Can you work these out from the model? Positions are in its coordinate system, mm. Coordinates: 2 decimals unless noted, no trailing zeros. Order: outer loops, then holes, each group sorted by start corner. A loop starts at its lowest first (then second) coordinate and runs counter-clockwise, first axis right, second up. Notation, with made-up numbers: (21.5, 18.5) -> (72.5, 18.5) arc R12 cw to (72.5, 40.5) -> close; hole circle Ø1 at (-35.5, 32.5). An arc over 180 degrees is marked (long way). Answer in a Markdown table with one row per item.
```python
from build123d import *

# Parameters (mm, degrees)
CYLINDER_R        = 35
CYLINDER_DEPTH    = 375
CYLINDER001_R     = 7.5
CYLINDER001_DEPTH = 390


with BuildPart() as part:
    # Cylinder → Cylinder (join)
    with BuildSketch(Plane.XY):
        Circle(CYLINDER_R)
    cylinder = extrude(amount=CYLINDER_DEPTH)

    # Cylinder001 → Cylinder001 (join)
    with BuildSketch(Plane.XY):
        Circle(CYLINDER001_R)
    cylinder001 = extrude(amount=CYLINDER001_DEPTH)

    # Mirrored001: Cylinder, Cylinder001 across XY
    add(cylinder.mirror(Plane.XY))
    add(cylinder001.mirror(Plane.XY))


solid = part.part
```
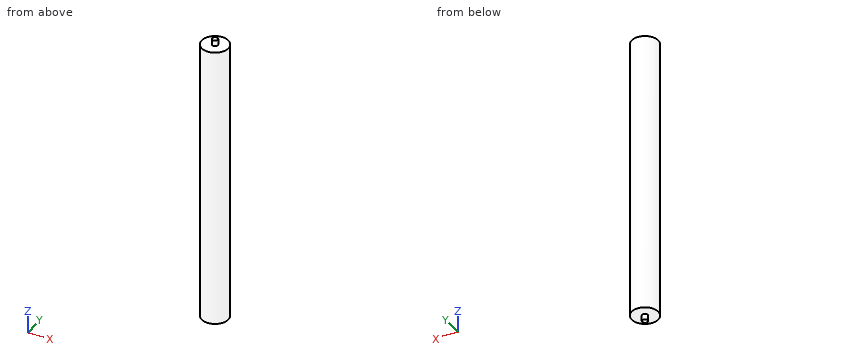
(1) Suppose I cut it at C-C (z = 202). Please give me the cut outline in (x, y).
Response values:
| item | result |
|---|---|
| outline | circle Ø70 at (0, 0) |
(2) Suppose I cut it at A-A (x = 0). Please give me the cut outline in (y, z), and give its area (4 significant figures).
Response values:
| item | result |
|---|---|
| outline | (-35, -375) -> (-7.5, -375) -> (-7.5, -390) -> (7.5, -390) -> (7.5, -375) -> (35, -375) -> (35, 375) -> (7.5, 375) -> (7.5, 390) -> (-7.5, 390) -> (-7.5, 375) -> (-35, 375) -> close |
| area | 52,950 mm2 |
(3) I need wall thicknesses on line 1 (Z direction, x = 28.5, y = 6); line 2 (Y direction, x = 1, z = 89.5); line 3 (X direction, y = 0.5, z = -269). Which ranges of each line are inside material? Lowest first, please. Write a range as [from, to].
Response values:
| item | result |
|---|---|
| line 1 | [-375, 375] |
| line 2 | [-34.99, 34.99] |
| line 3 | [-35, 35] |
(4) Suppose I cut it at D-D (y = -28.5). Please give me the cut outline in (x, z).
Response values:
| item | result |
|---|---|
| outline | (-20.32, -375) -> (20.32, -375) -> (20.32, 375) -> (-20.32, 375) -> close |
(5) Will these pins go through, and if not, where does the flat tip stop? pin 1 Ø8 at (x, y) = (-13, 1.5) entering from -Z; pin 2 Ø2 at (x, y) = (-3.5, -13) entering from +Z; pin 3 Ø3 at (y, z) = (-0.5, -7.5) entering from -X; pin 4 Ø6 at (x, z) = (-20.5, -137.5) entering from -Y.
Response values:
| item | result |
|---|---|
| pin 1 | z = -375 |
| pin 2 | z = 375 |
| pin 3 | x = -35 |
| pin 4 | y = -30.31 |
